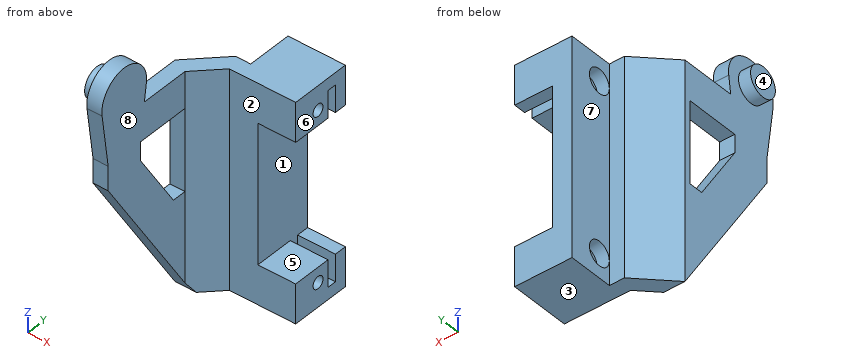
from build123d import *

# Parameters (mm, degrees)
EXTRUDE_1_DEPTH     = 18
CUT_EXTRUDE_1_REACH = 33.788
CUT_EXTRUDE_2_DEPTH = 6.25
SKETCH_4_R          = 1
CUT_EXTRUDE_3_DEPTH = 39.303882092
SKETCH_5_R          = 2
CUT_EXTRUDE_4_DEPTH = 2
EXTRUDE_3_DEPTH     = 2.5
EXTRUDE_START       = -2.5
SKETCH_6_3_R        = 2.5
EXTRUDE_4_DEPTH     = 2


with BuildPart() as part:
    # 草图1 → 凸台-拉伸1 (new, symmetric)
    with BuildSketch(Plane.XY):
        Polygon((0, 0), (0, 10), (-9.5, 10), (-9.5, 2.5), (-12, 2.5), (-17.5, -3), (-17.5, -19.5), (-15, -19.5), (-15, -4.035533906), (-10.964466094, 0), align=None)
    extrude(amount=EXTRUDE_1_DEPTH, both=True)

    # 草图2 → 切除-拉伸1 (cut, up to next)
    with BuildSketch(Plane.ZY.offset(17.5), mode=Mode.PRIVATE) as cut_extrude_1_sk1:
        Polygon((-1.5, -6.364922728), (-1.5, -4.035533906), (12, -4.035533906), (12, -13.035533906), (9.011266099, -13.035533906), align=None)
    cut_extrude_1_tool1 = extrude(cut_extrude_1_sk1.sketch, amount=-CUT_EXTRUDE_1_REACH, mode=Mode.PRIVATE) & part.part
    # 草图2 → 切除-拉伸1 (cut, up to next)
    with BuildSketch(Plane.ZY.offset(17.5), mode=Mode.PRIVATE) as cut_extrude_1_sk2:
        Polygon((-18, -3), (8, -19.5), (-18, -19.5), align=None)
    cut_extrude_1_tool2 = extrude(cut_extrude_1_sk2.sketch, amount=-CUT_EXTRUDE_1_REACH, mode=Mode.PRIVATE) & part.part
    add(cut_extrude_1_tool1.solids().sort_by_distance((-17.5, -7.612266, 6.566584))[0], mode=Mode.SUBTRACT)
    add(cut_extrude_1_tool2.solids().sort_by_distance((-17.5, -14, -9.333333))[0], mode=Mode.SUBTRACT)

    # 草图3 → 切除-拉伸2 (cut, symmetric)
    with BuildSketch(Plane(origin=(0, 8.894521129, 0.833176928), x_dir=(0, -1, 0), z_dir=(-1, 0, 0))):
        Polygon((2.394521129, 15.166823072), (2.394521129, 10.666823072), (8.894521129, 10.666823072), (8.894521129, -12.333176928), (2.394521129, -12.333176928), (2.394521129, -16.833176928), (0.894521129, -16.833176928), (0.894521129, -12.333176928), (-3.105478871, -12.333176928), (-3.105478871, 10.666823072), (0.894521129, 10.666823072), (0.894521129, 15.166823072), align=None)
    extrude(amount=CUT_EXTRUDE_2_DEPTH, both=True, mode=Mode.SUBTRACT)

    # 草图4 → 切除-拉伸3 (cut, through all)
    with BuildSketch(Plane(origin=(0, 8.894521129, 0.833176928), x_dir=(0, -1, 0), z_dir=(-1, 0, 0))):
        with Locations(Location((4.394521129, -14.833176928, 0), (0, 0, 180))):
            Circle(SKETCH_4_R)
        with Locations(Location((4.394521129, 13.166823072, 0), (0, 0, 180))):
            Circle(SKETCH_4_R)
    extrude(amount=CUT_EXTRUDE_3_DEPTH, mode=Mode.SUBTRACT)

    # 草图5 → 切除-拉伸4 (cut)
    with BuildSketch(Plane.ZY.offset(9.5)):
        with Locations(Location((14, 4.5, 0), (0, 0, 270))):
            Circle(SKETCH_5_R)
        with Locations(Location((-14, 4.5, 0), (0, 0, 270))):
            Circle(SKETCH_5_R)
    extrude(amount=-CUT_EXTRUDE_4_DEPTH, mode=Mode.SUBTRACT)

    # 草图6 → 凸台-拉伸3 (add)
    with BuildSketch(Plane(origin=(-15, 0, 0), x_dir=(0, 0, -1), z_dir=(1, 0, 0))):
        with BuildLine():
            ThreePointArc((-20.886363636, -11.809802124), (-26, -16.267766953), (-20.886363636, -20.725731782))
            Line((-20.886363636, -20.725731782), (-11.98162869, -19.5))
            Line((-11.98162869, -19.5), (-18, -19.5))
            Line((-18, -19.5), (-18, -12.207108463))
            Line((-18, -12.207108463), (-20.886363636, -11.809802124))
        make_face()
    extrude(amount=-EXTRUDE_3_DEPTH)

    # 草图6<3> → 凸台-拉伸4 (add)
    with BuildSketch(Plane(origin=(-15, 0, 0), x_dir=(0, 0, -1), z_dir=(1, 0, 0)).offset(EXTRUDE_START)):
        with Locations(Location((-21.5, -16.267766953, 0), (0, 0, 90))):
            Circle(SKETCH_6_3_R)
    extrude(amount=-EXTRUDE_4_DEPTH)


solid = part.part
Geometry check sheet. Reference: the model listing, model coordinates, mm. Face numbers are marked on the shaded views. A direction names the side the tool comes from. Give positions to 0.01 mm unless a question says otherwise; leave off trailing zeros. Order: outer loops, then holes, each group sorted by start corner. A loop starts at its lowest first (then second) coordinate and runs counter-clockwise, first axis right, second up. Notation, with made-up numbers: M 5.25,78.5 L 41.25,78.5 A19 ccw 41.25,94.5 Z; hole C 12,30.5 d11. An arc over 180 degrees is marked long. Use a Markdown table: item, result.
Item 1: Section check B-B (z = 9.5). Record the cut outline in (x, y), and give its area (3 significant figures).
Answers follow:
| item | result |
|---|---|
| outline | M -17.5,-19.5 L -15,-19.5 L -15,-13.04 L -17.5,-13.04 Z; M -17.5,-4.04 L -15,-4.04 L -10.96,0 L -6.25,0 L -6.25,10 L -9.5,10 L -9.5,2.5 L -12,2.5 L -17.5,-3 Z |
| area | 71.8 mm2 |
Item 2: Section check C-C (y = 4.5). Record the cut outline in (x, z), and give its area (3 significant figures).
Answers follow:
| item | result |
|---|---|
| outline | M -9.5,-18 L 0,-18 L 0,-15 L -7.5,-15 L -7.5,-16 L -9.5,-16 Z; M -9.5,-12 L -7.5,-12 L -7.5,-13 L 0,-13 L 0,-11.5 L -6.25,-11.5 L -6.25,11.5 L 0,11.5 L 0,13 L -7.5,13 L -7.5,12 L -9.5,12 Z; M -9.5,16 L -7.5,16 L -7.5,15 L 0,15 L 0,18 L -9.5,18 Z |
| area | 152 mm2 |
Item 3: Material ranges on line 1 along Z through (x, y) = (-9, 4.5); line 2 along Y through (x, z) = (-6, -14); line 3 along Z through (x, y) = (-1.25, 4.5), recorded low to high.
Answers follow:
| item | result |
|---|---|
| line 1 | z = -18 to -16, -12 to 12, 16 to 18 |
| line 2 | y = 0 to 3.5, 5.5 to 6.5, 8 to 10 |
| line 3 | z = -18 to -15, -13 to -11.5, 11.5 to 13, 15 to 18 |
Item 4: Section check A-A (x = -2.75). Record the cut outline in (y, z), and give its area (3 significant figures).
Answers follow:
| item | result |
|---|---|
| outline | M 0,-18 L 10,-18 L 10,-11.5 L 8,-11.5 L 8,-16 L 6.5,-16 L 6.5,-11.5 L 0,-11.5 Z; M 0,11.5 L 6.5,11.5 L 6.5,16 L 8,16 L 8,11.5 L 10,11.5 L 10,18 L 0,18 Z; hole C 4.5,-14 d2; hole C 4.5,14 d2 |
| area | 110 mm2 |
Item 5: Draft check along Z on the marked faces 1, 2 and 3. Enter one of: +Z half, -Z half, draft (parallel to the pull), parting line (faces both ways), or undercut.
Answers follow:
| item | result |
|---|---|
| face 1 | undercut |
| face 2 | draft |
| face 3 | -Z half |
Item 6: Depth check by flat-ended pin: P1, Ø9, axis at x = -3.5, z = -1.5, coming from the -Y side; P2, Ø2, axis at y = -17, z = 4.5, coming from the +X side; P3, Ø1.2, axis at x = -16.5, y = -8, coming from the -Z side. Enter the tip coordinate at first touch or a pass-through.
Answers follow:
| item | result |
|---|---|
| P1 | stops at y = 0 |
| P2 | stops at x = -15 |
| P3 | stops at z = -11.07 |
Item 7: Tool access check on the marked faces 4, 5, 6, 7 and 8. Record the directions out of +Z, -Z, +X, -X, +Y, -Y that give a thin tool (end or side, any length) a straight path to the whole face; none if there is none.
Answers follow:
| item | result |
|---|---|
| face 4 | +Z, -Z, -X, +Y, -Y |
| face 5 | +X, +Y, -Y |
| face 6 | +Z, -Z, +X, +Y, -Y |
| face 7 | +Z, -Z, -X, +Y |
| face 8 | +Z, -Z, +X, -Y |
Item 8: Section check D-D (x = -16). Record the cut outline in (y, z), and give its area (3 significant figures).
Answers follow:
| item | result |
|---|---|
| outline | M -20.73,20.89 L -19.5,11.98 L -19.5,8 L -3,-18 L -1.5,-18 L -1.5,18 L -12.21,18 L -11.81,20.89 A4.5 ccw long Z; hole M -13.04,9.01 L -6.36,-1.5 L -4.04,-1.5 L -4.04,12 L -13.04,12 Z |
| area | 411 mm2 |
